Input: part model. Units: mm. Frame: model coordinates. Face numbers are marked on the shaded views. Round coordinates to 2 decimals unless told otherwise and drop trailing zeros. Write each loop counter-clockwise with the first axis right and the second up, starting at its lowest first coordinate (ties: lowest second). Pieces come first, ordered by that corner, then holes. Notation, with made-up numbers: (58, -0.75) -> (106, -0.75) arc R28 ccw to (106, 23.25) -> close; hole circle Ø11 at (-19, 41). An arc over 180 degrees is marked (long way). Use CSV: the item, a comma, the result in double quotes.
```python
from build123d import *

# Parameters (mm, degrees)
SKETCH1_W           = 56.3
SKETCH1_H           = 71
BOSS_EXTRUDE1_DEPTH = 5.6
CUT_EXTRUDE1_DEPTH  = 1.6
SKETCH3_R           = 1.5
CUT_EXTRUDE2_DEPTH  = 4
SKETCH5_R           = 1.5
CUT_EXTRUDE3_DEPTH  = 4


with BuildPart() as part:
    # Sketch1 → Boss-Extrude1 (new body)
    with BuildSketch(Plane(origin=(0, 0, 0), x_dir=(1, 0, 0), z_dir=(0, 1, 0))):
        Rectangle(SKETCH1_W, SKETCH1_H)
    extrude(amount=BOSS_EXTRUDE1_DEPTH)

    # Sketch2 → Cut-Extrude1 (cut)
    with BuildSketch(Plane(origin=(0, 5.6, 0), x_dir=(1, 0, 0), z_dir=(0, 1, 0))):
        Polygon((26.65, -34), (-26.65, -34), (-26.65, 31), (-13.35, 31), (-10.35, 34), (21.65, 34), (24.65, 31), (26.65, 31), align=None)
    extrude(amount=-CUT_EXTRUDE1_DEPTH, mode=Mode.SUBTRACT)

    # Sketch3 → Cut-Extrude2 (cut)
    with BuildSketch(Plane(origin=(0, 4, 0), x_dir=(1, 0, 0), z_dir=(0, 1, 0))):
        with Locations(Location((-8.35, 31.5, 0), (0, 0, 270))):
            Circle(SKETCH3_R)
        with Locations(Location((19.65, 31.5, 0), (0, 0, 270))):
            Circle(SKETCH3_R)
        with Locations(Location((-23.85, -19, 0), (0, 0, 270))):
            Circle(SKETCH3_R)
    extrude(amount=-CUT_EXTRUDE2_DEPTH, mode=Mode.SUBTRACT)

    # Sketch5 → Cut-Extrude3 (cut)
    with BuildSketch(Plane(origin=(0, 4, 0), x_dir=(1, 0, 0), z_dir=(0, 1, 0))):
        with Locations(Location((-13, 17, 0), (0, 0, 270))):
            Circle(SKETCH5_R)
        with Locations(Location((13, -17, 0), (0, 0, 270))):
            Circle(SKETCH5_R)
        with Locations(Location((13, 17, 0), (0, 0, 270))):
            Circle(SKETCH5_R)
        with Locations(Location((-13, -17, 0), (0, 0, 270))):
            Circle(SKETCH5_R)
    extrude(amount=-CUT_EXTRUDE3_DEPTH, mode=Mode.SUBTRACT)


solid = part.part
```
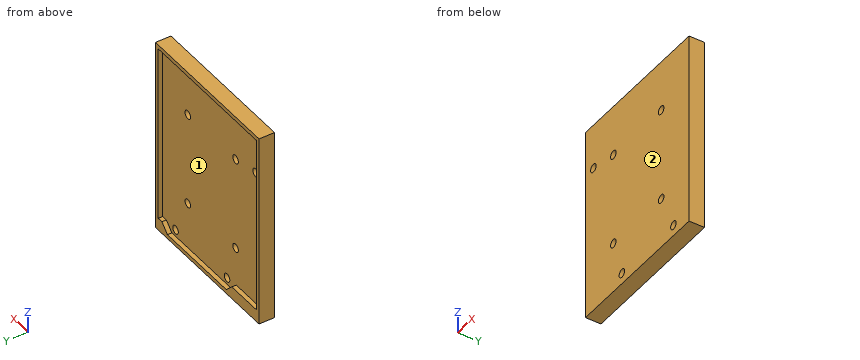
Item 1: Section query A-A on x = 19.65. Return the cut outline in (y, z).
Worked answers:
outline,"(0, -35.5) -> (5.6, -35.5) -> (5.6, -34) -> (4, -34) -> (4, -33) -> (0, -33) -> close; (0, -30) -> (4, -30) -> (4, 34) -> (5.6, 34) -> (5.6, 35.5) -> (0, 35.5) -> close"
Item 2: Section query D-D on x = -23.85. Return the cut outline in (y, z).
Worked answers:
outline,"(0, -35.5) -> (5.6, -35.5) -> (5.6, -31) -> (4, -31) -> (4, 17.5) -> (0, 17.5) -> close; (0, 20.5) -> (4, 20.5) -> (4, 34) -> (5.6, 34) -> (5.6, 35.5) -> (0, 35.5) -> close"
Item 3: First-contact query: pin 1 Ø4 at (x, z) = (19.65, -31.5) entering from +Y; pin 2 Ø10 at (x, z) = (-11.5, 7.5) entering from -Y; pin 3 Ø1.8 at (x, z) = (-23.85, 19) entering from -Y. Flat tips, straight axial feed; report the tip coordinate or a pass-through.
Worked answers:
pin 1,"stops at y = 4"
pin 2,"stops at y = 0"
pin 3,"passes through"
Item 4: Line query: line 1 (X direction, y = 2.9, z = -31.5); line 2 (X direction, y = 1.05, z = -17); line 3 (Z direction, x = 9, y = 5.4). Output: solid intervals per line, ascending.
Worked answers:
line 1,"x = -28.15 to -9.85, -6.85 to 18.15, 21.15 to 28.15"
line 2,"x = -28.15 to -14.5, -11.5 to 11.5, 14.5 to 28.15"
line 3,"z = -35.5 to -34, 34 to 35.5"
Item 5: Pull-direction query (Z, two-part tool) for the marked faces 1 and 2; classes: +Z half, -Z half, draft (parallel to the pull), parting line (faces both ways), or undercut.
Worked answers:
face 1,"undercut"
face 2,"draft"
Item 6: Section query C-C on z = -6. Return the cut outline in (x, y).
Worked answers:
outline,"(-28.15, 0) -> (28.15, 0) -> (28.15, 5.6) -> (26.65, 5.6) -> (26.65, 4) -> (-26.65, 4) -> (-26.65, 5.6) -> (-28.15, 5.6) -> close"
Item 7: Section query B-B on z = -17. Return the cut outline in (x, y).
Worked answers:
outline,"(-28.15, 0) -> (-14.5, 0) -> (-14.5, 4) -> (-26.65, 4) -> (-26.65, 5.6) -> (-28.15, 5.6) -> close; (-11.5, 0) -> (11.5, 0) -> (11.5, 4) -> (-11.5, 4) -> close; (14.5, 0) -> (28.15, 0) -> (28.15, 5.6) -> (26.65, 5.6) -> (26.65, 4) -> (14.5, 4) -> close"
